Work out the finished part from the listing and answer in its coordinate system (mm). Round coordinates to 2 decimals unless told otherwise and drop trailing zeros. Loops run counter-clockwise (first coordinate to the right, second up) from the corner with the lowest first, then second, coordinate; pieces in that order, holes last.
```python
from build123d import *

# Parameters (mm, degrees)
F0_W      = 50
F0_H      = 100
F1_DEPTH  = 3
F2_W      = 3
F2_H      = 25
F3_DEPTH  = 3
F4_R      = 30
F5_R      = 5
F6_R      = 5
F7_R      = 7.5
F8_DEPTH  = 3
F9_R      = 7.5
F10_DEPTH = 25


with BuildPart() as f1:
    # F0 (on Right) → F1 (new body)
    with BuildSketch(Plane.YZ):
        with Locations((-103.739034, 70.985424)):
            Rectangle(F0_W, F0_H)
    extrude(amount=F1_DEPTH)

    # F2 (on face) → F3 (cut)
    with BuildSketch(Plane.YZ.offset(3)):
        with Locations((-90.239034, 70.224934)):
            Rectangle(F2_W, F2_H)
    extrude(amount=-F3_DEPTH, mode=Mode.SUBTRACT)

    # F4
    f4_edges = [f1.edges().sort_by_distance(p)[0] for p in [
        (1.5, -128.739034, 120.985424),
    ]]
    fillet(f4_edges, radius=F4_R)

    # F5
    f5_edges = [f1.edges().sort_by_distance(p)[0] for p in [
        (1.5, -78.739034, 120.985424),
    ]]
    fillet(f5_edges, radius=F5_R)

    # F6
    f6_edges = [f1.edges().sort_by_distance(p)[0] for p in [
        (1.5, -128.739034, 20.985424),
    ]]
    fillet(f6_edges, radius=F6_R)

    # F7 (on face) → F8 (cut)
    with BuildSketch(Plane.YZ.offset(3)):
        with Locations((-113.739034, 95.985424)):
            Circle(F7_R)
    extrude(amount=-F8_DEPTH, mode=Mode.SUBTRACT)

    # F9 (on face) → F10 (cut)
    with BuildSketch(Plane.YZ.offset(3)):
        with Locations((-108.739034, 45.985424)):
            Circle(F9_R)
    extrude(amount=-F10_DEPTH, mode=Mode.SUBTRACT)


solid = f1.part
```
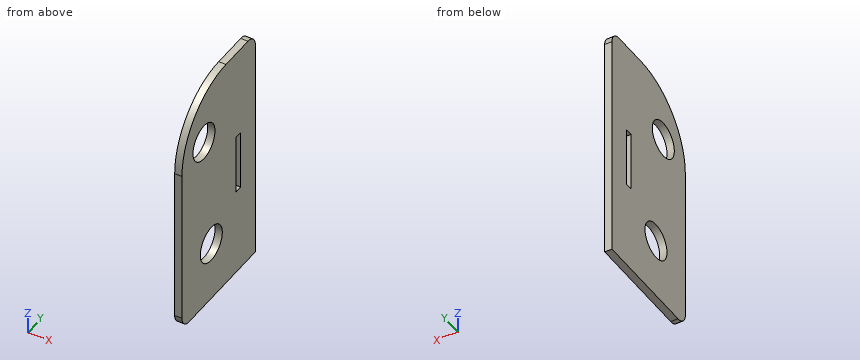
1. Consider probe 1 along Z at (x, y) = (2.8, -90.5); probe 2 along Z at (x, y) = (2.3, -108); probe 3 along Y at (x, z) = (1.2, 65). Determine where each line is inside the solid, lowest interval first.
Answer key:
probe 1: z = 20.99 to 57.72, 82.72 to 120.99
probe 2: z = 20.99 to 38.52, 53.45 to 91.16, 100.81 to 119.52
probe 3: y = -128.74 to -91.74, -88.74 to -78.74
2. Given pin 1 (1 mm diameter, centred on x = 1.5, y = -101, fed in from +Z), flat-ended and moving along its own axis, determine where the tip first touches the part or whether it passes through.
Answer key:
pin 1: stops at z = 120.93
3. Find section C-C (x = 2.5). Write down the section's boundary in (y, z), then the cut area to 3 significant figures.
Answer key:
outline: (-128.74, 25.99) arc R5 ccw to (-123.74, 20.99) - (-78.74, 20.99) - (-78.74, 115.99) arc R5 ccw to (-83.74, 120.99) - (-98.74, 120.99) arc R30 ccw to (-128.74, 90.99) - close; hole circle Ø15 at (-113.74, 95.99); hole circle Ø15 at (-108.74, 45.99); hole (-91.74, 57.72) - (-88.74, 57.72) - (-88.74, 82.72) - (-91.74, 82.72) - close
area: 4,370 mm2
4. Find section B-B (y = -107.5). Write down the section's boundary in (x, z), then the cut area to 3 significant figures.
Answer key:
outline: (0, 20.99) - (3, 20.99) - (3, 38.59) - (0, 38.59) - close; (0, 53.38) - (3, 53.38) - (3, 91.82) - (0, 91.82) - close; (0, 100.15) - (3, 100.15) - (3, 119.68) - (0, 119.68) - close
area: 227 mm2
5. Find section A-A (z = 64). Write down the section's boundary in (x, y).
Answer key:
outline: (0, -128.74) - (3, -128.74) - (3, -91.74) - (0, -91.74) - close; (0, -88.74) - (3, -88.74) - (3, -78.74) - (0, -78.74) - close
6. Find section D-D (z = 40.5). Write down the section's boundary in (x, y).
Answer key:
outline: (0, -128.74) - (3, -128.74) - (3, -113.85) - (0, -113.85) - close; (0, -103.62) - (3, -103.62) - (3, -78.74) - (0, -78.74) - close
